CAD build for the part. Positions are in the model's coordinates, mm. Face numbers are marked on the shaded views. A direction names the side the tool comes from. Coordinates: 2 decimals unless noted, no trailing zeros. Order: outer loops, then holes, each group sorted by start corner. A loop starts at its lowest first (then second) coordinate and runs counter-clockwise, first axis right, second up. Notation, with made-up numbers: M 32,22 L 88,22 A26 ccw 88,46 Z; hole C 87.5,36.5 d11. An arc over 180 degrees is marked long. Write item = value, one per line. Start each with the question number.
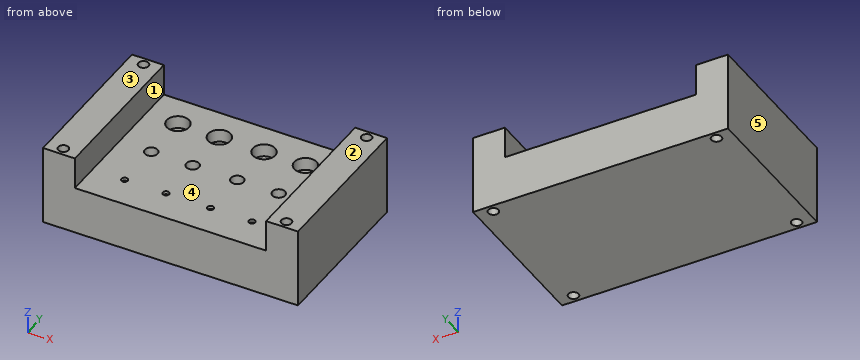
```python
from build123d import *

# Parameters (mm, degrees)
F0_W     = 60
F0_H     = 50
F0_R     = 1
F0_R_2   = 2
F0_R_3   = 3.5
F0_W_2   = 10
F0_R_4   = 1.6
F1_DEPTH = 15
F2_DEPTH = 10
F3_DEPTH = 4
F4_DEPTH = 3
F5_DEPTH = 1


with BuildPart() as f1:
    # F0 (on Top) → F1 (new body)
    with BuildSketch(Plane.XY):
        Rectangle(F0_W, F0_H)
        with Locations((-20, -15)):
            Circle(F0_R, mode=Mode.SUBTRACT)
        with Locations((-7, -15)):
            Circle(F0_R, mode=Mode.SUBTRACT)
        with Locations((7, -15)):
            Circle(F0_R, mode=Mode.SUBTRACT)
        with Locations((20, -15)):
            Circle(F0_R, mode=Mode.SUBTRACT)
        with Locations((-20, 0)):
            Circle(F0_R_2, mode=Mode.SUBTRACT)
        with Locations((-7, 0)):
            Circle(F0_R_2, mode=Mode.SUBTRACT)
        with Locations((-20, 15)):
            Circle(F0_R_3, mode=Mode.SUBTRACT)
        with Locations((-7, 15)):
            Circle(F0_R_3, mode=Mode.SUBTRACT)
        with Locations((7, 0)):
            Circle(F0_R_2, mode=Mode.SUBTRACT)
        with Locations((20, 0)):
            Circle(F0_R_2, mode=Mode.SUBTRACT)
        with Locations((7, 15)):
            Circle(F0_R_3, mode=Mode.SUBTRACT)
        with Locations((20, 15)):
            Circle(F0_R_3, mode=Mode.SUBTRACT)
        with Locations((-35, 0)):
            Rectangle(F0_W_2, F0_H)
        with Locations((-35, -22.5)):
            Circle(F0_R_4, mode=Mode.SUBTRACT)
        with Locations((-35, 22.5)):
            Circle(F0_R_4, mode=Mode.SUBTRACT)
        with Locations((35, 0)):
            Rectangle(F0_W_2, F0_H)
        with Locations((35, -22.5)):
            Circle(F0_R_4, mode=Mode.SUBTRACT)
        with Locations((35, 22.5)):
            Circle(F0_R_4, mode=Mode.SUBTRACT)
        with Locations((-20, 15)):
            Circle(F0_R_3)
        with Locations((-7, 15)):
            Circle(F0_R_3)
        with Locations((7, 15)):
            Circle(F0_R_3)
        with Locations((20, 15)):
            Circle(F0_R_3)
        with Locations((7, 0)):
            Circle(F0_R_2)
        with Locations((20, 0)):
            Circle(F0_R_2)
        with Locations((-7, 0)):
            Circle(F0_R_2)
        with Locations((-20, 0)):
            Circle(F0_R_2)
        with Locations((-20, -15)):
            Circle(F0_R)
        with Locations((-7, -15)):
            Circle(F0_R)
        with Locations((7, -15)):
            Circle(F0_R)
        with Locations((20, -15)):
            Circle(F0_R)
    extrude(amount=-F1_DEPTH)

    # F0 (on Top) → F2 (join)
    with BuildSketch(Plane.XY):
        with Locations((-35, 0)):
            Rectangle(F0_W_2, F0_H)
        with Locations((-35, -22.5)):
            Circle(F0_R_4, mode=Mode.SUBTRACT)
        with Locations((-35, 22.5)):
            Circle(F0_R_4, mode=Mode.SUBTRACT)
        with Locations((35, 0)):
            Rectangle(F0_W_2, F0_H)
        with Locations((35, -22.5)):
            Circle(F0_R_4, mode=Mode.SUBTRACT)
        with Locations((35, 22.5)):
            Circle(F0_R_4, mode=Mode.SUBTRACT)
    extrude(amount=F2_DEPTH)

    # F0 (on Top) → F3 (cut)
    with BuildSketch(Plane.XY):
        with Locations((-20, 15)):
            Circle(F0_R_3)
        with Locations((-7, 15)):
            Circle(F0_R_3)
        with Locations((7, 15)):
            Circle(F0_R_3)
        with Locations((20, 15)):
            Circle(F0_R_3)
    extrude(amount=-F3_DEPTH, mode=Mode.SUBTRACT)

    # F0 (on Top) → F4 (cut)
    with BuildSketch(Plane.XY):
        with Locations((-20, 0)):
            Circle(F0_R_2)
        with Locations((-7, 0)):
            Circle(F0_R_2)
        with Locations((7, 0)):
            Circle(F0_R_2)
        with Locations((20, 0)):
            Circle(F0_R_2)
    extrude(amount=-F4_DEPTH, mode=Mode.SUBTRACT)

    # F0 (on Top) → F5 (cut)
    with BuildSketch(Plane.XY):
        with Locations((-20, -15)):
            Circle(F0_R)
        with Locations((-7, -15)):
            Circle(F0_R)
        with Locations((7, -15)):
            Circle(F0_R)
        with Locations((20, -15)):
            Circle(F0_R)
    extrude(amount=-F5_DEPTH, mode=Mode.SUBTRACT)


solid = f1.part
```
1. Slice it at B-B (y = 22.5). Write the cut outline in (x, z).
2. Slice it at C-C (x = 7). Write the cut outline in (y, z).
3. Flat gauge pins, fed straight in: pin 1 (5 mm diameter, centred on x = 17, y = 17, fed in from +Z); pin 2 (1.2 mm diameter, centred on x = 7.5, y = -0.5, fed in from +Z); pin 3 (1.6 mm diameter, centred on x = -7, y = -15, fed in from +Z). Where does each tip first touch, or does it go through?
4. Mould opens along X. For the marked faces 3, 4 and 5 say: released by +X, released by -X, zero draft, split by the parting line, or undercut.
5. 3-axis set-ups, long thin cutter, end or side, ignore diameter. For the marked faces 1 and 2: which of +Z, -Z, +X, -X, +Y, -Y reach the whole face in a straight line?
6. Slice it at D-D (y = 0). Write the cut outline in (x, z).
7. Slice it at A-A (z = 4.5). Write the cut outline in (x, y).
8. Probe L1, parallel to Y at x = -7, z = -1.5; L2, parallel to Y at x = 35, z = -8; L3, parallel to Y at x = 20, z = -0.3. List the from-to ranges inside material, lowest first.
Calculated:
q1.outline = M -40,-15 L -36.6,-15 L -36.6,10 L -40,10 Z; M -33.4,-15 L 33.4,-15 L 33.4,10 L 30,10 L 30,0 L -30,0 L -30,10 L -33.4,10 Z; M 36.6,-15 L 40,-15 L 40,10 L 36.6,10 Z
q2.outline = M -25,-15 L 25,-15 L 25,0 L 18.5,0 L 18.5,-4 L 11.5,-4 L 11.5,0 L 2,0 L 2,-3 L -2,-3 L -2,0 L -14,0 L -14,-1 L -16,-1 L -16,0 L -25,0 Z
q3.pin_1 = 0
q3.pin_2 = -3
q3.pin_3 = -1
q4.face_3 = zero draft
q4.face_4 = undercut
q4.face_5 = released by -X
q5.face_1 = +Z, +Y, -Y
q5.face_2 = +Z, +X, -X, +Y, -Y
q6.outline = M -40,-15 L 40,-15 L 40,10 L 30,10 L 30,0 L 22,0 L 22,-3 L 18,-3 L 18,0 L 9,0 L 9,-3 L 5,-3 L 5,0 L -5,0 L -5,-3 L -9,-3 L -9,0 L -18,0 L -18,-3 L -22,-3 L -22,0 L -30,0 L -30,10 L -40,10 Z
q7.outline = M -40,-25 L -30,-25 L -30,25 L -40,25 Z; M 30,-25 L 40,-25 L 40,25 L 30,25 Z; hole C -35,-22.5 d3.2; hole C -35,22.5 d3.2; hole C 35,-22.5 d3.2; hole C 35,22.5 d3.2
q8.L1 = -25 to -2, 2 to 11.5, 18.5 to 25
q8.L2 = -25 to -24.1, -20.9 to 20.9, 24.1 to 25
q8.L3 = -25 to -16, -14 to -2, 2 to 11.5, 18.5 to 25
